```python
from build123d import *

# Parameters (mm, degrees)
MGN7H_START                                 = 33.9
MGN7H_30_8_X_17_MM_BLOCK_PROFILE_W          = 30.8
MGN7H_30_8_X_17_MM_BLOCK_PROFILE_H          = 17
MGN7H_30_8_X_17_MM_BLOCK_DEPTH              = 6.5
RAIL_START                                  = 33.85
RAIL_SLOT_AND_RUNNING_CLEARANCE_PROFILE_W   = 31
RAIL_SLOT_AND_RUNNING_CLEARANCE_PROFILE_H   = 7.5
RAIL_SLOT_AND_RUNNING_CLEARANCE_DEPTH       = 3.6
NOMINAL_START                               = 34.45
NOMINAL_RACEWAY_SHOULDERS_PROFILE_W         = 30.8
NOMINAL_RACEWAY_SHOULDERS_PROFILE_H         = 0.65
NOMINAL_RACEWAY_SHOULDERS_DEPTH             = 0.8
M2_START                                    = 37.9
M2_X_2_5_BLOCK_HOLES_13_X_12_MM_PITCH_PR_R  = 0.8
M2_X_2_5_BLOCK_HOLES_13_X_12_MM_PITCH_DEPTH = 2.6


with BuildPart() as part:
    # MGN7H 30.8 x 17 mm block profile → MGN7H 30.8 x 17 mm block (new body)
    with BuildSketch(Plane.XY.offset(MGN7H_START)):
        with Locations((8.5, 19)):
            Rectangle(MGN7H_30_8_X_17_MM_BLOCK_PROFILE_W, MGN7H_30_8_X_17_MM_BLOCK_PROFILE_H)
    extrude(amount=MGN7H_30_8_X_17_MM_BLOCK_DEPTH)

    # Rail slot and running clearance profile → Rail slot and running clearance (cut)
    with BuildSketch(Plane.XY.offset(RAIL_START)):
        with Locations((8.5, 19)):
            Rectangle(RAIL_SLOT_AND_RUNNING_CLEARANCE_PROFILE_W, RAIL_SLOT_AND_RUNNING_CLEARANCE_PROFILE_H)
    extrude(amount=RAIL_SLOT_AND_RUNNING_CLEARANCE_DEPTH, mode=Mode.SUBTRACT)

    # Nominal raceway shoulders profile → Nominal raceway shoulders (add)
    with BuildSketch(Plane.XY.offset(NOMINAL_START)):
        with Locations((8.5, 15.475)):
            Rectangle(NOMINAL_RACEWAY_SHOULDERS_PROFILE_W, NOMINAL_RACEWAY_SHOULDERS_PROFILE_H)
        with Locations((8.5, 22.525)):
            Rectangle(NOMINAL_RACEWAY_SHOULDERS_PROFILE_W, NOMINAL_RACEWAY_SHOULDERS_PROFILE_H)
    extrude(amount=NOMINAL_RACEWAY_SHOULDERS_DEPTH)

    # M2 x 2.5 block holes 13 x 12 mm pitch profile → M2 x 2.5 block holes 13 x 12 mm pitch (cut)
    with BuildSketch(Plane.XY.offset(M2_START)):
        with Locations((2, 13)):
            Circle(M2_X_2_5_BLOCK_HOLES_13_X_12_MM_PITCH_PR_R)
        with Locations((2, 25)):
            Circle(M2_X_2_5_BLOCK_HOLES_13_X_12_MM_PITCH_PR_R)
        with Locations((15, 13)):
            Circle(M2_X_2_5_BLOCK_HOLES_13_X_12_MM_PITCH_PR_R)
        with Locations((15, 25)):
            Circle(M2_X_2_5_BLOCK_HOLES_13_X_12_MM_PITCH_PR_R)
    extrude(amount=M2_X_2_5_BLOCK_HOLES_13_X_12_MM_PITCH_DEPTH, mode=Mode.SUBTRACT)


solid = part.part
```
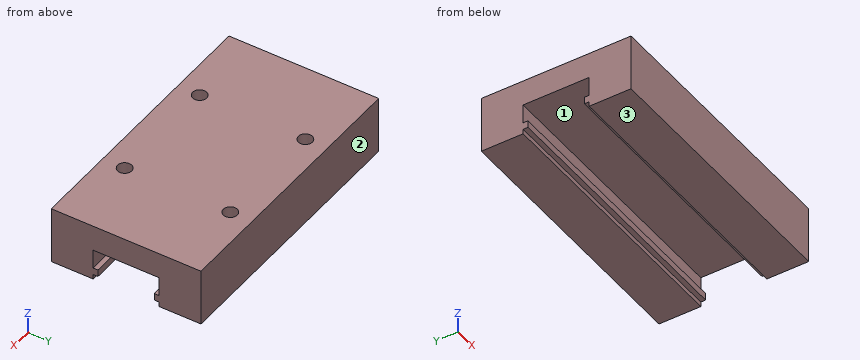
For this review, take the finished solid that the model builds, in its own axes (mm). Face numbers are marked on the shaded views. Round coordinates to 2 decimals unless told otherwise and drop trailing zeros. Write each loop counter-clockwise with the first axis right and the second up, starting at its lowest first coordinate (ties: lowest second). Pieces come first, ordered by that corner, then holes. Notation, with made-up numbers: M 41.5,16.5 L 85.5,16.5 A20 ccw 85.5,41.5 Z; hole C -37,34.5 d1. An arc over 180 degrees is marked long. One line per item, written item: value. Start each with the question number.
(1) We need section B-B (y = 13). Give the boundary of the cut face in (x, z), and give its area (3 significant figures).
(2) We need section C-C (z = 36). Give the boundary of the cut face in (x, y).
(3) We need section A-A (z = 39.75). Give the boundary of the cut face in (x, y).
(4) We need section D-D (x = 2). Give the boundary of the cut face in (y, z), and give its area (3 significant figures).
(5) Wall thickness on line 1 (Y direction, x = 15, z = 38.7); line 2 (X direction, y = 25, z = 38.4); line 3 (Y direction, x = 10, z = 34.75): over which ranges is each line inside the solid? List them lowest first.
(6) The part is to be moulded in two halves that separate along Y. For the marked faces 1, 2 and 3, say which applies: released by +Y, released by -Y, zero draft, split by the parting line, or undercut.
(7) Insertion check: pin 1 (0.5 mm diameter, centred on x = 2, y = 25, fed in from +Z). The pin has a flat end and moves straight along its axis. Give the tip position at first contact, or say it passes through.
Result:
1. outline: M -6.9,33.9 L 23.9,33.9 L 23.9,40.4 L 15.8,40.4 L 15.8,37.9 L 14.2,37.9 L 14.2,40.4 L 2.8,40.4 L 2.8,37.9 L 1.2,37.9 L 1.2,40.4 L -6.9,40.4 Z
1. area: 192 mm²
2. outline: M -6.9,10.5 L 23.9,10.5 L 23.9,15.25 L -6.9,15.25 Z; M -6.9,22.75 L 23.9,22.75 L 23.9,27.5 L -6.9,27.5 Z
3. outline: M -6.9,10.5 L 23.9,10.5 L 23.9,27.5 L -6.9,27.5 Z; hole C 2,13 d1.6; hole C 2,25 d1.6; hole C 15,13 d1.6; hole C 15,25 d1.6
4. outline: M 10.5,33.9 L 15.25,33.9 L 15.25,34.45 L 15.8,34.45 L 15.8,35.25 L 15.25,35.25 L 15.25,37.45 L 22.75,37.45 L 22.75,35.25 L 22.2,35.25 L 22.2,34.45 L 22.75,34.45 L 22.75,33.9 L 27.5,33.9 L 27.5,40.4 L 25.8,40.4 L 25.8,37.9 L 24.2,37.9 L 24.2,40.4 L 13.8,40.4 L 13.8,37.9 L 12.2,37.9 L 12.2,40.4 L 10.5,40.4 Z
4. area: 76.8 mm²
5. line 1: 10.5 to 12.2, 13.8 to 24.2, 25.8 to 27.5
5. line 2: -6.9 to 1.2, 2.8 to 14.2, 15.8 to 23.9
5. line 3: 10.5 to 15.8, 22.2 to 27.5
6. face 1: undercut
6. face 2: released by +Y
6. face 3: zero draft
7. pin 1: z = 37.9
